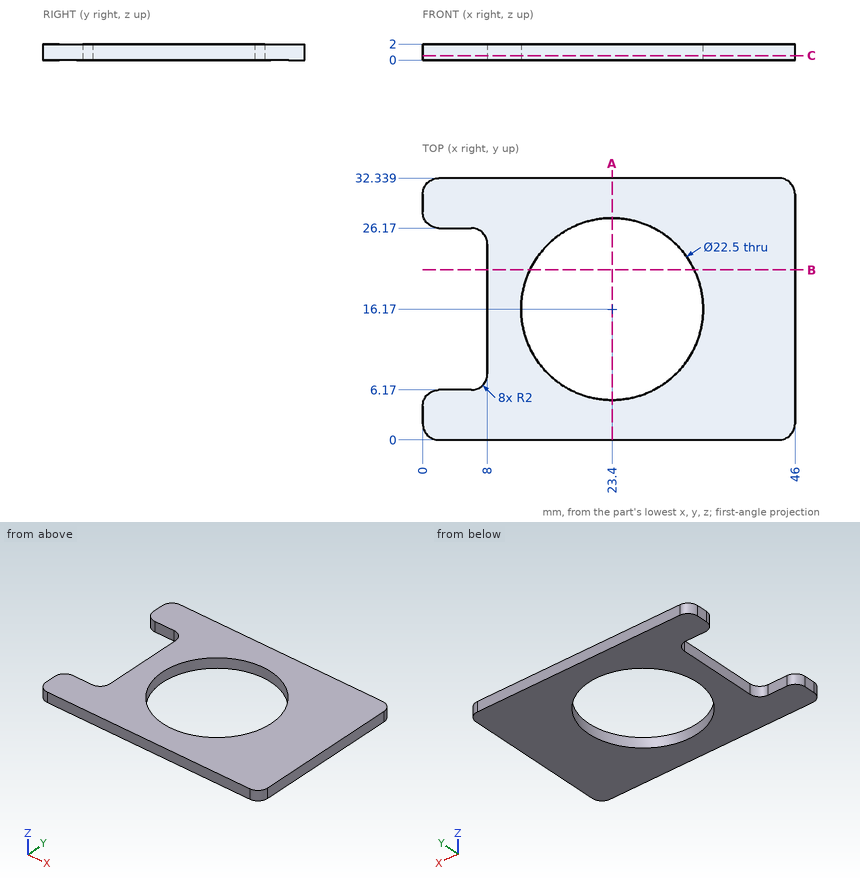
Study the drawing (mm; zero at the part's minimum x, y, z) and answer. Round coordinates to 2 decimals unless told otherwise and drop trailing zeros. Loops run counter-clockwise (first coordinate to the right, second up) from the corner with the lowest first, then second, coordinate; pieces in that order, holes last.
Q1. Section C-C, the plane z = 0.55 is taken. Determine the outline of the cut face in (x, y).
Q2. Find the intervals of material crossed by line 1 (Y direction, x = 4.5, z = 0.25); line 2 (Y direction, x = 23.4, z = 0.65); line 3 (X direction, y = 7, z = 0.1) (1 decimal), in increasing order.
Q3. Section B-B, the plane y = 21 is taken. Determine the outline of the cut face in (x, z).
Q4. Section A-A, the plane x = 23.4 is taken. Determine the outline of the cut face in (y, z), then the cut area to 3 significant figures.
Q5. Given pin 1 Ø1 at (y, z) = (19, 0.5) entering from -X, flat-ended and moving along its own axis, determine where the tip first touches the part or whether it passes through.
Completed:
1. outline: (0, 2) arc R2 ccw to (2, 0) - (44, 0) arc R2 ccw to (46, 2) - (46, 30.34) arc R2 ccw to (44, 32.34) - (2, 32.34) arc R2 ccw to (0, 30.34) - (0, 28.17) arc R2 ccw to (2, 26.17) - (6, 26.17) arc R2 cw to (8, 24.17) - (8, 8.17) arc R2 cw to (6, 6.17) - (2, 6.17) arc R2 ccw to (0, 4.17) - close; hole circle Ø22.5 at (23.4, 16.17)
2. line 1: y = 0 to 6.17, 26.17 to 32.34
2. line 2: y = 0 to 4.92, 27.42 to 32.34
2. line 3: x = 7.6 to 16.9, 29.9 to 46
3. outline: (8, 0) - (13.24, 0) - (13.24, 2) - (8, 2) - close; (33.56, 0) - (46, 0) - (46, 2) - (33.56, 2) - close
4. outline: (0, 0) - (4.92, 0) - (4.92, 2) - (0, 2) - close; (27.42, 0) - (32.34, 0) - (32.34, 2) - (27.42, 2) - close
4. area: 19.7 mm2
5. pin 1: stops at x = 8
